Check sheet for the modelled part. Datum: model origin and axes. Units: mm. Give positions to 0.01 mm unless a question says otherwise; leave off trailing zeros. Write each loop counter-clockwise with the first axis right and the second up, starting at its lowest first coordinate (ties: lowest second). Pieces come first, ordered by that corner, then holes. Notation, with made-up numbers: (-18, 49) -> (27, 49) arc R33 cw to (27, 79) -> close; hole circle Ø11 at (46, 50). An arc over 180 degrees is marked (long way). Write each question's results on one line, items separated by ' | '. Start each with the question number.
```python
from build123d import *

# Parameters (mm, degrees)
F0_W     = 3.175
F0_H     = 12.7
F1_DEPTH = 44.45
F3_DEPTH = 3.176
F5_DEPTH = 82.55
F6_R     = 2.54


with BuildPart() as f1:
    # F0 (on Front) → F1 (new body, symmetric)
    with BuildSketch(Plane.XZ):
        Rectangle(F0_W, F0_H)
    extrude(amount=F1_DEPTH, both=True)

    # F2 (on face) → F3 (cut, through all)
    with BuildSketch(Plane.YZ.offset(1.5875)):
        Polygon((44.45, -6.35), (44.45, 3.175), (12.7, 2.54), (6.35, -6.35), align=None)
    extrude(amount=-F3_DEPTH, mode=Mode.SUBTRACT)

    # F4 (on face) → F5 (cut)
    with BuildSketch(Plane.XZ.offset(44.45)):
        Polygon((1.5875, -4.516913), (-1.5875, -6.35), (1.5875, -6.35), align=None)
    extrude(amount=-F5_DEPTH, mode=Mode.SUBTRACT)

    # F6
    f6_edges = [f1.edges().sort_by_distance(p)[0] for p in [
        (0, 12.7, 2.54),
    ]]
    fillet(f6_edges, radius=F6_R)


solid = f1.part
```
Item 1: Section check B-B on y = -35.5. Record the boundary of the cut face in (x, z), then the cut area to 3 significant figures.
Item 2: Section check C-C on z = -0.75. Record the boundary of the cut face in (x, y), then the cut area to 3 significant figures.
Item 3: Thickness scan on probe 1 along Y at (x, z) = (-0.95, 1.5); probe 2 along Y at (x, z) = (-0.6, 0); probe 3 along Z at (x, y) = (-0.95, 7.5). Record the ranges inside material, lowest first. Write a range as from..to.
Check sheet entries:
1) outline: (-1.59, -6.35) -> (1.59, -4.52) -> (1.59, 6.35) -> (-1.59, 6.35) -> close | area: 37.4 mm^2
2) outline: (-1.59, -44.45) -> (1.59, -44.45) -> (1.59, 10.35) -> (-1.59, 10.35) -> close | area: 174 mm^2
3) probe 1: y = -44.45..11.96 | probe 2: y = -44.45..10.89 | probe 3: z = -4.74..6.35
